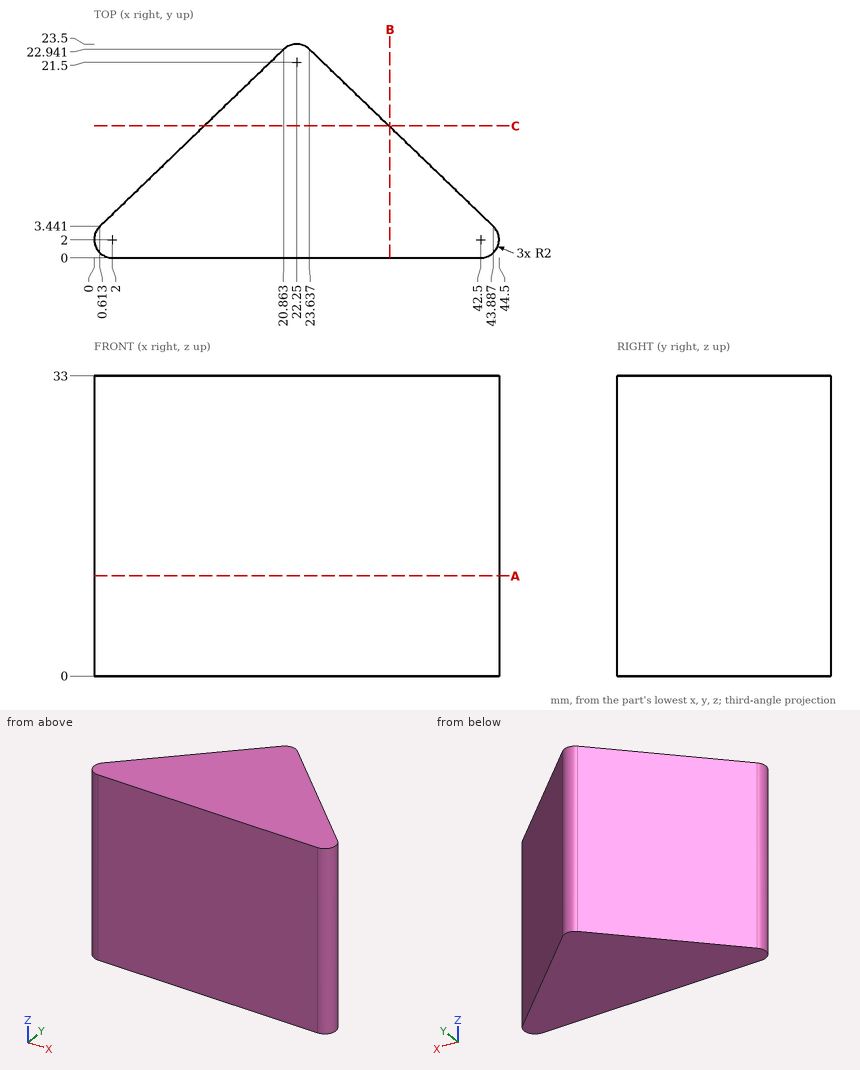
The drawing under review shows one solid part. Ordinate dimensions are in mm from its lowest x, y, z. Coordinates: 2 decimals unless noted, no trailing zeros. Order: outer loops, then holes, each group sorted by start corner. A loop starts at its lowest first (then second) coordinate and runs counter-clockwise, first axis right, second up. Notation, with made-up numbers: (-31, 84.25) -> (-2, 84.25) arc R17 ccw to (-2, 92.25) -> close; hole circle Ø6 at (-22, 88.5). An arc over 180 degrees is marked (long way). Return JSON: item names as keys, results as strings.
1. We need section B-B on x = 32.5. Write out the cut boundary in (y, z), and give its area (3 significant figures).
Answer block:
{"outline": "(0, 0) -> (14.41, 0) -> (14.41, 33) -> (0, 33) -> close", "area": "475 mm²"}
2. For line 1 (X direction, y = 8.5, z = 19) (1 decimal); line 2 (X direction, y = 18.75, z = 21.5); line 3 (Y direction, x = 29.5, z = 11.5) (1 decimal), list the stretches that pass through material, from the lowest coordinate up. Write a range as from..to.
Answer block:
{"line 1": "5.9..38.6", "line 2": "16.51..27.99", "line 3": "0..17.3"}
3. We need section C-C on y = 14.5. Write out the cut boundary in (x, z).
Answer block:
{"outline": "(12.1, 0) -> (32.4, 0) -> (32.4, 33) -> (12.1, 33) -> close"}
4. We need section A-A on z = 11. Write out the cut boundary in (x, y).
Answer block:
{"outline": "(0.61, 3.44) arc R2 ccw to (2, 0) -> (42.5, 0) arc R2 ccw to (43.89, 3.44) -> (23.64, 22.94) arc R2 ccw to (20.86, 22.94) -> close"}
5. For pin 1 Ø12 at (x, z) = (13, 5) entering from +Y; pin 2 Ø1 at (x, z) = (23.5, 17) entering from +Y; pin 3 Ø3 at (y, z) = (13.5, 20.5) entering from -X, all flat-tipped, find the tip position at first contact; note any pin that passes through.
Answer block:
{"pin 1": "y = 21.15", "pin 2": "y = 23.35", "pin 3": "x = 9.5"}
